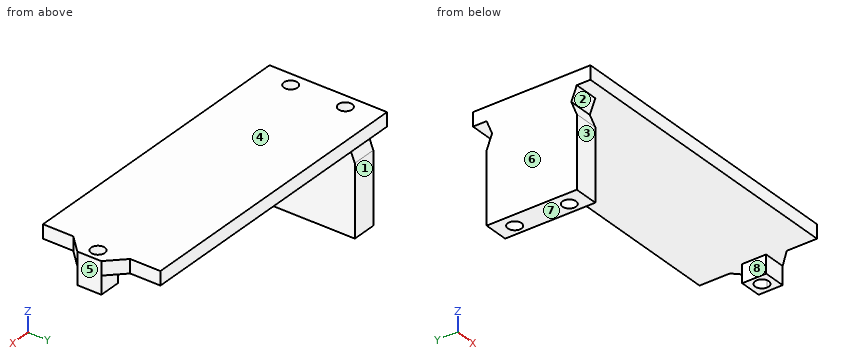
```python
from build123d import *
from build123d.topology import SkipClean

# Parameters (mm, degrees)
SKETCH1_R           = 1.5875
BOSS_EXTRUDE1_DEPTH = 3.175
BOSS_EXTRUDE2_START = -22.86
SKETCH1_3_W         = 5.715
SKETCH1_3_H         = 20.955
SKETCH1_3_R         = 1.5875
BOSS_EXTRUDE2_DEPTH = 22.86
BOSS_EXTRUDE3_START = -4.191
BOSS_EXTRUDE3_DEPTH = 4.191
CHAMFER1_SIZE       = 3.81
SKETCH3_W           = 69.85
SKETCH3_H           = 3.175
BOSS_EXTRUDE4_DEPTH = 3.175
CUT_EXTRUDE6_DEPTH  = 76.639668991


with BuildPart() as part:
    # Sketch1 → Boss-Extrude1 (new body)
    with BuildSketch(Plane.XY):
        Polygon((0, 20.955), (-69.85, 20.955), (-69.85, 0), (0, 0), (0, 7.6835), (3.81, 7.6835), (3.81, 13.2715), (0, 13.2715), align=None)
        with Locations((-66.675, 16.8275)):
            Circle(SKETCH1_R, mode=Mode.SUBTRACT)
        with Locations((-66.675, 4.1275)):
            Circle(SKETCH1_R, mode=Mode.SUBTRACT)
        with Locations((1.143, 10.4775)):
            Circle(SKETCH1_R, mode=Mode.SUBTRACT)
    extrude(amount=BOSS_EXTRUDE1_DEPTH)

    # Sketch1<3> → Boss-Extrude2 (add)
    with BuildSketch(Plane.XY.offset(BOSS_EXTRUDE2_START)):
        with Locations((-66.9925, 10.4775)):
            Rectangle(SKETCH1_3_W, SKETCH1_3_H)
        with Locations((-66.675, 4.1275)):
            Circle(SKETCH1_3_R, mode=Mode.SUBTRACT)
        with Locations((-66.675, 16.8275)):
            Circle(SKETCH1_3_R, mode=Mode.SUBTRACT)
    extrude(amount=BOSS_EXTRUDE2_DEPTH)

    # Sketch1<4> → Boss-Extrude3 (add)
    with SkipClean():  # the faces are left unmerged after this step: merging them gives an invalid solid
        with BuildSketch(Plane.XY.offset(BOSS_EXTRUDE3_START)):
            with BuildLine():
                Line((3.81, 13.2715), (0, 13.2715))
                Line((0, 13.2715), (0, 11.579183825))
                ThreePointArc((0, 11.579183825), (1.73698811, 11.949686936), (2.7305, 10.4775))
                ThreePointArc((2.7305, 10.4775), (1.73698811, 9.005313064), (0, 9.375816175))
                Line((0, 9.375816175), (0, 7.6835))
                Line((0, 7.6835), (3.81, 7.6835))
                Line((3.81, 7.6835), (3.81, 13.2715))
            make_face()
            with BuildLine():
                Line((0, 11.579183825), (0, 13.2715))
                Line((0, 13.2715), (-1.27, 13.2715))
                Line((-1.27, 13.2715), (-1.27, 7.6835))
                Line((-1.27, 7.6835), (0, 7.6835))
                Line((0, 7.6835), (0, 9.375816175))
                ThreePointArc((0, 9.375816175), (-0.4445, 10.4775), (0, 11.579183825))
            make_face()
        extrude(amount=BOSS_EXTRUDE3_DEPTH)

    # Chamfer1
    # the kernel refuses this chamfer: 3.81 mm, written as the material it adds along each edge
    with BuildSketch(Plane(origin=(0, 7.6835, 0), x_dir=(-0.027495876610586462, -0.9996219169112968, 0), z_dir=(0, 0, 1))) as chamfer1_piece_1_section:
        Polygon((CHAMFER1_SIZE * 0.999621916911, CHAMFER1_SIZE * 0.0274958766106), (-CHAMFER1_SIZE * 0.0274958766106, CHAMFER1_SIZE * 0.999621916911), (0, 0), align=None)
    chamfer1_piece_1 = extrude(amount=3.175, mode=Mode.PRIVATE)
    chamfer1_piece_1 = split(chamfer1_piece_1, bisect_by=Plane(origin=(3.81, 6.424660172, 1.5875), z_dir=(-1, 0, 0)), keep=Keep.TOP, mode=Mode.PRIVATE)
    add(chamfer1_piece_1)
    with BuildSketch(Plane(origin=(0, 13.2715, 0), x_dir=(-0.027495876610586452, 0.9996219169112968, 0), z_dir=(0, 0, 1))) as chamfer1_piece_2_section:
        Polygon((CHAMFER1_SIZE * 0.999621916911, -CHAMFER1_SIZE * 0.0274958766106), (-CHAMFER1_SIZE * 0.0274958766106, -CHAMFER1_SIZE * 0.999621916911), (0, 0), align=None)
    chamfer1_piece_2 = extrude(amount=3.175, mode=Mode.PRIVATE)
    chamfer1_piece_2 = split(chamfer1_piece_2, bisect_by=Plane(origin=(3.81, 14.530339828, 1.5875), z_dir=(-1, 0, 0)), keep=Keep.TOP, mode=Mode.PRIVATE)
    add(chamfer1_piece_2)

    # Sketch3 → Boss-Extrude4 (add)
    with BuildSketch(Plane(origin=(0, 20.955, 0), x_dir=(1, 0, 0), z_dir=(0, 1, 0))):
        with Locations((-34.925, -1.5875)):
            Rectangle(SKETCH3_W, SKETCH3_H)
    boss_extrude4 = extrude(amount=BOSS_EXTRUDE4_DEPTH)

    # Mirror1: Boss-Extrude4 across plane
    add(boss_extrude4.mirror(Plane(origin=(0, 10.4775, 0), x_dir=(0, 0, 1), z_dir=(0, -1, 0))))

    # Sketch6 → Cut-Extrude6 (cut, through all)
    with BuildSketch(Plane(origin=(-64.135, 0, 0), x_dir=(0, 0, -1), z_dir=(1, 0, 0))):
        Polygon((0, 20.955), (3.175, 19.685), (6.35, 20.955), align=None)
        Polygon((3.175, 1.27), (6.35, 0), (0, 0), align=None)
    extrude(amount=-CUT_EXTRUDE6_DEPTH, mode=Mode.SUBTRACT)


solid = part.part
```
Here's how the part is built. I have some questions about the finished solid (model axes, mm). Face numbers are marked on the shaded views. A direction names the side the tool comes from. Coordinates: 2 decimals unless noted, no trailing zeros. Order: outer loops, then holes, each group sorted by start corner. A loop starts at its lowest first (then second) coordinate and runs counter-clockwise, first axis right, second up. Notation, with made-up numbers: M 70.25,31.25 L 96.25,31.25 A23 ccw 96.25,65.25 Z; hole C -9.5,-16 d7. An arc over 180 degrees is marked long. Answer as a JSON object with one key per item and string values. Group by question number.
(1) Suppose I cut it at B-B, the plane x = -52. Please give me the cut outline in (y, z) (3 decimals), then the cut area to 3 significant figures.
(2) For pin 1 (5.5 mm diameter, centred on x = 1.5, y = 11, fed in from -Z); pin 2 (3 mm diameter, centred on x = -65.5, z = -16.5, fed in from -Y); pin 3 (4 mm diameter, centred on x = -3.5, y = 6, fed in from -Z), each with a flat end and sliding along its axis, tell me the tip position at first contact or that it passes through.
(3) If we mould it in two halves opening along X, with no side actions, what happens to the marked faces 5, 6, 7 and 8? For each: released by +X, released by -X, zero draft, split by the parting line, or undercut.
(4) Suppose I cut it at D-D, the plane y = -0.75. Please give me the cut outline in (x, z) (3 decimals).
(5) Which directions (+Z, -Z, +X, -X, +Y, -Y) give clear straight access to the entire face, cutting with the end or side of a thin tool? Please do the marked faces 1, 2, 3 and 4.
(6) Suppose I cut it at A-A, the plane z = 1. State how many separate pieces and enclosed holes the cut face has, then the cut area to 3 significant figures.
(7) I need wall thicknesses on probe 1 along X at (y, z) = (10.5, 0.25); probe 2 along Z at (x, y) = (-38, 17.75) (3 decimals); probe 3 along X at (y, z) = (10, -1.75) (3 decimals). Which ranges of each line are inside material? Lowest first, please.
Values found:
{
 "1": {"outline": "M -3.175,0 L 24.13,0 L 24.13,3.175 L -3.175,3.175 Z", "area": "86.7 mm^2"},
 "2": {"pin 1": "stops at z = -4.19", "pin 2": "stops at y = 0", "pin 3": "stops at z = 0"},
 "3": {"face 5": "released by +X", "face 6": "released by -X", "face 7": "zero draft", "face 8": "undercut"},
 "4": {"outline": "M -69.85,0 L 0,0 L 0,3.175 L -69.85,3.175 Z"},
 "5": {"face 1": "-Z, +X, -X, +Y", "face 2": "+X, -X, -Y", "face 3": "-Z, +X, -X, -Y", "face 4": "+Z, +X, -X, +Y, -Y"},
 "6": {"separate pieces": "1", "enclosed holes": "3", "area": "1,920 mm^2"},
 "7": {"probe 1": "x = -69.85 to -0.44, 2.73 to 3.81", "probe 2": "z = 0 to 3.175", "probe 3": "x = -69.85 to -64.135, -1.27 to -0.371, 2.657 to 3.81"}
}
